from build123d import *

# Parameters (mm, degrees)
F0_R     = 7
F0_R_2   = 5.5
F1_DEPTH = 4
F2_R     = 7
F3_DEPTH = 2
F4_SIZE  = 1.5
F5_SIZE  = 0.3


with BuildPart() as f1:
    # F0 (on Top) → F1 (new body)
    with BuildSketch(Plane.XY):
        Circle(F0_R)
        Circle(F0_R_2, mode=Mode.SUBTRACT)
    extrude(amount=F1_DEPTH)

    # F2 (on face) → F3 (join)
    with BuildSketch(Plane(origin=(0, 0, 0), x_dir=(1, 0, 0), z_dir=(0, 0, -1))):
        Circle(F2_R)
    extrude(amount=F3_DEPTH)

    # F4
    f4_edges = [f1.edges().sort_by_distance(p)[0] for p in [
        (-7, 0, -2),
    ]]
    chamfer(f4_edges, length=F4_SIZE)

    # F5
    f5_edges = [f1.edges().sort_by_distance(p)[0] for p in [
        (-5.5, 0, 4),
    ]]
    chamfer(f5_edges, length=F5_SIZE)


solid = f1.part
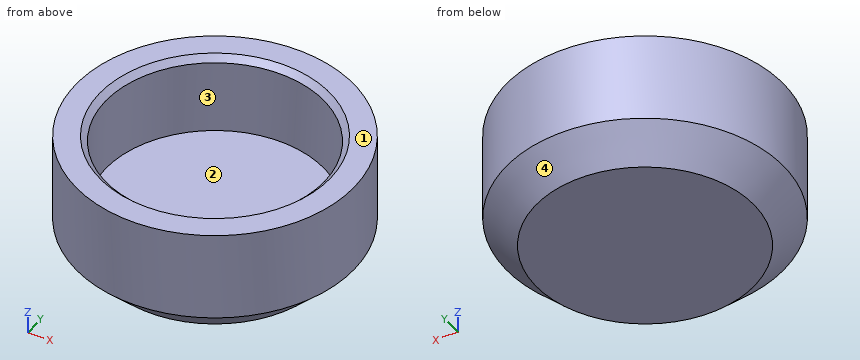
Geometry: final body of the model. Coordinates: model frame, mm. Face numbers are marked on the shaded views. Coordinates: 2 decimals unless noted, no trailing zeros. Order: outer loops, then holes, each group sorted by start corner. A loop starts at its lowest first (then second) coordinate and runs counter-clockwise, first axis right, second up. Notation, with made-up numbers: M 39,16.25 L 53,16.25 A30 ccw 53,42.25 Z; hole C 14.5,87 d7. An arc over 180 degrees is marked long. One line per question, with ' | ' between items. Start each with the question number.
Item 1: Pin query (flat end, axial travel): pin 1 Ø4 at (x, y) = (1, 5.5) entering from +Z; pin 2 Ø1.5 at (x, z) = (5.5, -1) entering from -Y; pin 3 Ø1 at (x, z) = (-3.5, 1.5) entering from +Y; pin 4 Ø1.5 at (x, y) = (-1.5, -3) entering from +Z. Return the tip coordinate at first contact, or that it passes through.
Item 2: Ray query, probe 1 along Y at (x, z) = (0, 2.85); probe 2 along Z at (x, y) = (-0.5, 2.75); probe 3 along X at (y, z) = (-2.5, 2.7). Return the intervals inside material, ascending. Write a range as [from, to].
Item 3: Cut plane C-C, the plane z = -1.5. Return the cut outline in (x, y).
Item 4: Draft query along X for the marked faces 1, 2, 3 and 4. Return one class per face: released by +X, released by -X, zero draft, split by the parting line, or undercut.
Item 5: Cut plane A-A, the plane x = 0. Return the cut outline in (y, z), then the cut area to 3 significant figures.
A:
1) pin 1: stops at z = 4 | pin 2: stops at y = -4.96 | pin 3: stops at y = 6.32 | pin 4: stops at z = 0
2) probe 1: y = [-7, -5.5], [5.5, 7] | probe 2: z = [-2, 0] | probe 3: x = [-6.54, -4.9], [4.9, 6.54]
3) outline: C 0,0 d12
4) face 1: zero draft | face 2: undercut | face 3: undercut | face 4: split by the parting line
5) outline: M -7,-0.5 L -5.5,-2 L 5.5,-2 L 7,-0.5 L 7,4 L 5.8,4 L 5.5,3.7 L 5.5,0 L -5.5,0 L -5.5,3.7 L -5.8,4 L -7,4 Z | area: 37.7 mm2
